```python
from build123d import *

# Parameters (mm, degrees)
F2_DEPTH = 28.4
F3_DEPTH = 4
F6_D     = 5
F6_DEPTH = 5
F6_TIP   = 1.5021515476
F7_D     = 5
F7_DEPTH = 7
F7_TIP   = 1.5021515476
F8_R     = 1


with BuildPart() as f2:
    # F0 (on Front) → F2 (new body)
    with BuildSketch(Plane.XZ):
        with BuildLine():
            Line((23.6029717884, 8.2401288069), (37.7647548615, 13.1842060911))
            ThreePointArc((37.7647548615, 13.1842060911), (30.9779974122, 25.3054080451), (20.4548362885, 34.3744043208))
            Line((20.4548362885, 34.3744043208), (12.7842726803, 21.4840027005))
            ThreePointArc((12.7842726803, 21.4840027005), (19.3612483826, 15.8158800282), (23.6029717884, 8.2401288069))
        make_face()
    extrude(amount=F2_DEPTH)

    # F1 (on Front) + F0 (on Front) → F3 (join)
    with BuildSketch(Plane.XZ):
        with BuildLine():
            ThreePointArc((15.2340019476, 15.8721512297), (17.0378985767, 13.9179744248), (18.5928148308, 11.7604097152))
            Line((18.5928148308, 11.7604097152), (21.4911474241, 12.7722583124))
            ThreePointArc((21.4911474241, 12.7722583124), (22.6606475272, 10.5591218219), (23.6029717884, 8.2401288069))
            Line((23.6029717884, 8.2401288069), (37.7647548615, 13.1842060911))
            ThreePointArc((37.7647548615, 13.1842060911), (30.9779974122, 25.3054080451), (20.4548362885, 34.3744043208))
            Line((20.4548362885, 34.3744043208), (12.7842726803, 21.4840027005))
            ThreePointArc((12.7842726803, 21.4840027005), (14.8685909795, 20.0978855177), (16.8038497839, 18.5102845046))
            Line((16.8038497839, 18.5102845046), (15.2340019476, 15.8721512297))
        make_face()
    with BuildSketch(Plane.XZ):
        with BuildLine():
            Line((23.6029717884, 8.2401288069), (37.7647548615, 13.1842060911))
            ThreePointArc((37.7647548615, 13.1842060911), (30.9779974122, 25.3054080451), (20.4548362885, 34.3744043208))
            Line((20.4548362885, 34.3744043208), (12.7842726803, 21.4840027005))
            ThreePointArc((12.7842726803, 21.4840027005), (19.3612483826, 15.8158800282), (23.6029717884, 8.2401288069))
        make_face()
    extrude(amount=-F3_DEPTH)

    # F6 (one way)
    with BuildSketch(Plane(origin=(29.109795575, 0, 23.7793052059), x_dir=(0, 1, 0), z_dir=(-0.7744499353, 0, -0.6326352011))):
        with Locations((-5, 0)):
            Circle(F6_D / 2)
    extrude(amount=-F6_DEPTH, mode=Mode.SUBTRACT)
    with Locations(Plane(origin=(29.109795575, 0, 23.7793052059), x_dir=(0, 1, 0), z_dir=(-0.7744499353, 0, -0.6326352011))):
        with Locations((-5, 0)):
            with Locations((0, 0, -(F6_DEPTH + F6_TIP / 2))):  # 118° drill point
                Cone(0, F6_D / 2, F6_TIP, mode=Mode.SUBTRACT)

    # F7
    with Locations(Plane(origin=(29.109795575, 0, 23.7793052059), x_dir=(0, 1, 0), z_dir=(0.7744499353, 0, 0.6326352011))):
        with Locations((-5, 0)):
            Hole(F7_D / 2, depth=F7_DEPTH)
            with Locations((0, 0, -(F7_DEPTH + F7_TIP / 2))):  # 118° drill point
                Cone(0, F7_D / 2, F7_TIP, mode=Mode.SUBTRACT)

    # F8
    f8_edges = [f2.edges().sort_by_distance(p)[0] for p in [
        (21.491147, 2, 12.772258),
        (16.80385, 2, 18.510285),
    ]]
    fillet(f8_edges, radius=F8_R)


solid = f2.part
```
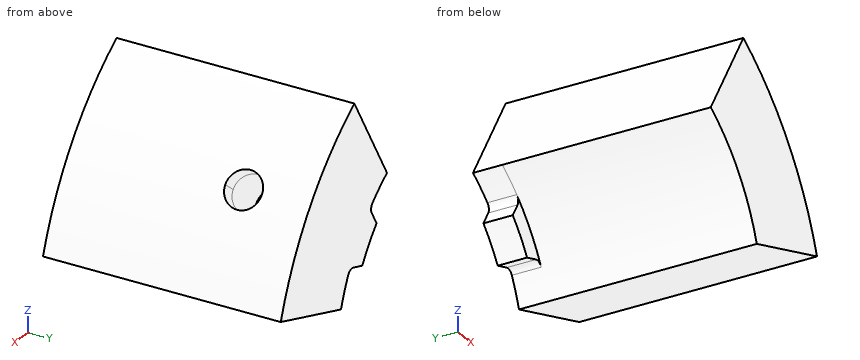
The listing builds one solid part. Answer for the finished solid, in the listing's coordinates (mm). Give positions to 0.01 mm unless a question says otherwise; leave off trailing zeros. Write each loop counter-clockwise with the first axis right and the second up, starting at its lowest first coordinate (ties: lowest second). Pieces come first, ordered by that corner, then holes. Notation, with made-up numbers: (-20, -26) - (6, -26) arc R23 ccw to (6, 7) - close; hole circle Ø8 at (46, 32). An arc over 180 degrees is marked (long way). Use one line per item in the form item = value. Start each with the question number.
1) Find section D-D on z = 17. Determine the outline of the cut face in (x, y), plus the area to 3 significant figures.
2) Find section C-C on z = 28.5. Determine the outline of the cut face in (x, y), plus the area to 3 significant figures.
3) Find section A-A on y = -15.5. Determine the outline of the cut face in (x, z), plus the area to 3 significant figures.
4) Consider line 1 along Y through (x, z) = (28, 24.25); line 2 along Z through (x, y) = (32.25, -3.5); line 3 along Z through (x, y) = (16.25, -13.5). Determine where each line is inside the solid, lowest interval first. Write a range as from..to.
5) Flat-ended cylindrical pins translate along their axes: pin 1 Ø8 at (y, z) = (-7.5, 31) entering from +X; pin 2 Ø5 at (y, z) = (-23.5, 20.5) entering from +X; pin 3 Ø12 at (x, y) = (23.5, -2.5) entering from +Z. Find the tip coordinate at first contact, or state that the pin passes through.
6) Find section B-B on x = 21.5. Determine the outline of the cut face in (y, z).
Geometry results:
q1.outline = (15.91, 0) - (18.33, 0) - (18.33, -28.4) - (36.21, -28.4) - (36.21, 4) - (15.91, 4) - close
q1.area = 589 mm2
q2.outline = (16.96, -28.4) - (28.07, -28.4) - (28.07, 4) - (16.96, 4) - close
q2.area = 360 mm2
q3.outline = (12.78, 21.48) arc R25 cw to (23.6, 8.24) - (37.76, 13.18) arc R40 ccw to (20.45, 34.37) - close
q3.area = 340 mm2
q4.line_1 = -28.4..-7.26, -2.74..4
q4.line_2 = 11.26..23.66
q4.line_3 = 19..27.31
q5.pin_1 = 29.51
q5.pin_2 = 35.72
q5.pin_3 = 34.37
q6.outline = (-28.4, 12.76) - (0, 12.76) - (0, 12.44) - (4, 12.44) - (4, 33.73) - (-28.4, 33.73) - close
